Geometry: see drawing. Coordinates: mm, zero at the bounding-box minimum. A direction names the side the tool comes from. Round coordinates to 2 decimals unless told otherwise and drop trailing zeros. Loops run counter-clockwise (first coordinate to the right, second up) from the corner with the lowest first, then second, coordinate; pieces in that order, holes last.
(1) Cut plane B-B, the plane x = 5. Output: boundary loops of the cut face in (y, z), and give its area (3 significant figures).
(2) Access query for the marked faces 1 and 2. Directions: +Z, -Z, +X, -X, +Y, -Y. A direction counts if a zero-diameter tool reaches every point of the face in a straight line with its end or side. Return the directions, or none.
(3) Cut plane D-D, the plane x = 8. Output: boundary loops of the cut face in (y, z).
(4) Line query: line 1 (Y direction, x = 2.5, z = 1); line 2 (Y direction, x = 1.5, z = 4.5); line 3 (X direction, y = 28.5, z = 8). Output: solid intervals per line, ascending.
(5) Cut plane C-C, the plane y = 48. Output: boundary loops of the cut face in (x, z), and give its area (3 significant figures).
(6) Cut plane A-A, the plane z = 5. Output: boundary loops of the cut face in (x, y).
(7) First-contact query: pin 1 Ø4 at (x, y) = (1, 7) entering from +Z; pin 2 Ø6 at (y, z) = (44.5, 1) entering from -X; pin 3 Ø3 at (x, z) = (5.5, 3.5) entering from -Y; pin 4 Ø5 at (x, y) = (7.5, 29) entering from +Z. Flat tips, straight axial feed; report the tip coordinate or a pass-through.
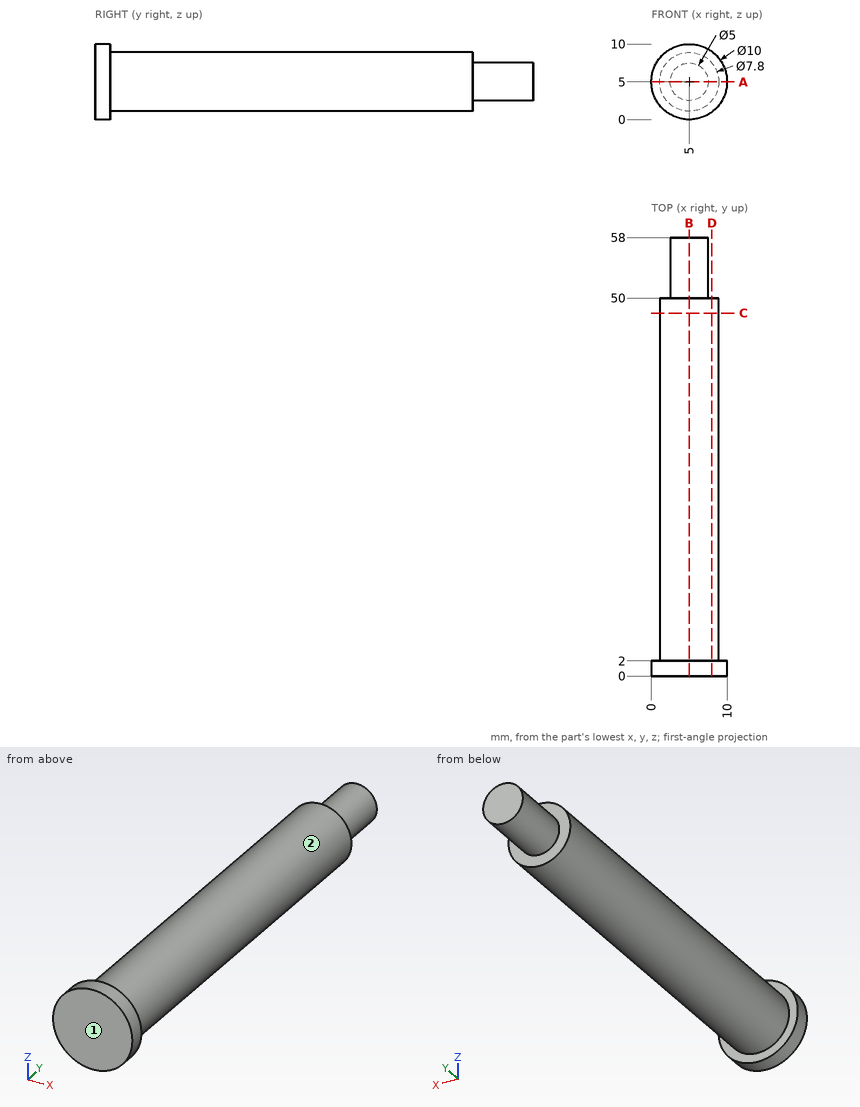
Reported:
1. outline: (0, 0) - (2, 0) - (2, 1.1) - (50, 1.1) - (50, 2.5) - (58, 2.5) - (58, 7.5) - (50, 7.5) - (50, 8.9) - (2, 8.9) - (2, 10) - (0, 10) - close
1. area: 434 mm2
2. face 1: +Z, -Z, +X, -X, -Y
2. face 2: +Y
3. outline: (0, 1) - (2, 1) - (2, 2.51) - (50, 2.51) - (50, 7.49) - (2, 7.49) - (2, 9) - (0, 9) - close
4. line 1: y = 0 to 2
4. line 2: y = 0 to 50
4. line 3: x = 2.51 to 7.49
5. outline: circle Ø7.8 at (5, 5)
5. area: 47.8 mm2
6. outline: (0, 0) - (10, 0) - (10, 2) - (8.9, 2) - (8.9, 50) - (7.5, 50) - (7.5, 58) - (2.5, 58) - (2.5, 50) - (1.1, 50) - (1.1, 2) - (0, 2) - close
7. pin 1: stops at z = 8.35
7. pin 2: stops at x = 1.23
7. pin 3: stops at y = 0
7. pin 4: stops at z = 8.9
